Source: CAD feature listing. Evaluate the final solid. Frame: model axes, mm. A direction names the side the tool comes from. Round coordinates to 2 decimals unless told otherwise and drop trailing zeros. Loops run counter-clockwise (first coordinate to the right, second up) from the corner with the lowest first, then second, coordinate; pieces in that order, holes last. Notation, with made-up numbers: (83, 55.25) - (105, 55.25) arc R18 cw to (105, 72.25) - close; hole circle Ø8 at (77.25, 67). An arc over 180 degrees is marked (long way). Use CSV: the item, a comma, the result in double quotes. Start each with the question number.
from build123d import *

# Parameters (mm, degrees)
F0_W     = 86
F0_H     = 66
F1_DEPTH = 2
F2_DEPTH = 10
F3_W     = 92
F3_H     = 72
F3_W_2   = 86
F3_H_2   = 66
F4_DEPTH = 4
F5_W     = 94
F5_H     = 74
F5_W_2   = 88
F5_H_2   = 2
F5_W_3   = 2
F5_H_3   = 68
F6_DEPTH = 2
F0_R     = 2.5
F7_DEPTH = 5


with BuildPart() as f1:
    # F0 (on Top) → F1 (new body)
    with BuildSketch(Plane.XY):
        Rectangle(F0_W, F0_H)
    extrude(amount=F1_DEPTH)

    # F0 (on Top) → F2 (join)
    with BuildSketch(Plane.XY):
        Polygon((47, -37), (47, 37), (5, 37), (-5, 37), (-47, 37), (-47, -37), align=None)
        Rectangle(F0_W, F0_H, mode=Mode.SUBTRACT)
    extrude(amount=F2_DEPTH)

    # F3 (on face) → F4 (cut)
    with BuildSketch(Plane.XY.offset(10)):
        Rectangle(F3_W, F3_H)
        Rectangle(F3_W_2, F3_H_2, mode=Mode.SUBTRACT)
    extrude(amount=-F4_DEPTH, mode=Mode.SUBTRACT)

    # F5 (on face) → F6 (join)
    with BuildSketch(Plane.XY.offset(10)):
        Rectangle(F5_W, F5_H)
        Polygon((-44, -36), (-46, -36), (-46, -34), (-46, 34), (-46, 36), (-44, 36), (44, 36), (46, 36), (46, 34), (46, -34), (46, -36), (44, -36), align=None, mode=Mode.SUBTRACT)
        with Locations((0, 35)):
            Rectangle(F5_W_2, F5_H_2)
        with Locations((0, -35)):
            Rectangle(F5_W_2, F5_H_2)
        with Locations((-45, 0)):
            Rectangle(F5_W_3, F5_H_3)
        with Locations((45, 0)):
            Rectangle(F5_W_3, F5_H_3)
        with Locations((-45, 35)):
            Rectangle(F5_W_3, F5_H_2)
        with Locations((45, 35)):
            Rectangle(F5_W_3, F5_H_2)
        with Locations((45, -35)):
            Rectangle(F5_W_3, F5_H_2)
        with Locations((-45, -35)):
            Rectangle(F5_W_3, F5_H_2)
    extrude(amount=F6_DEPTH)

    # F0 (on Top) → F7 (join)
    with BuildSketch(Plane.XY):
        with BuildLine():
            Line((-5, 37), (5, 37))
            Line((5, 37), (5, 47))
            ThreePointArc((5, 47), (0, 42), (-5, 47))
            Line((-5, 47), (-5, 37))
        make_face()
        with BuildLine():
            ThreePointArc((-5, 47), (0, 42), (5, 47))
            ThreePointArc((5, 47), (0, 52), (-5, 47))
        make_face()
        with Locations((0, 47)):
            Circle(F0_R, mode=Mode.SUBTRACT)
    extrude(amount=F7_DEPTH)


solid = f1.part
1. Section query A-A on x = 0. Return the cut outline in (y, z), and give its area (3 significant figures).
2. Section query D-D on x = 34.5. Return the cut outline in (y, z).
3. Reachability of faces 4 (the flat face through (-1, 33, 4)), 5 (the flat face through (5, 42, 2)), 6 (the flat face through (-5, 42, 2)) from +Z, -Z, +X, -X, +Y, -Y: full face, straight path, thin tool, end or side. Return the list, or none.
4. Contact query for flat-ended pins moving along their axis: P1, Ø4, axis at x = -23, y = 40, coming from the +Z side; P2, Ø0.6, axis at x = -14.5, z = 11.5, coming from the +Y side; P3, Ø1.5, axis at y = 42.5, z = 2.5, coming from the -X side. Output: stop coordinate, or through.
5. Section query C-C on y = -18. Return the cut outline in (x, z).
6. Line query: line 1 along X through (y, z) = (-13.5, 5); line 2 along Y through (x, z) = (7, 7.5); line 3 along X through (y, z) = (16.5, 11). Output: solid intervals per line, ascending.
7. Section query B-B on z = 7.25. Return the cut outline in (x, y).
8. Mould query, pull axis Z, two halves, no side actions, for faces 1 (the flat face through (0, 43, 5)), 2 (the flat face through (-1, -33, 4)), 3 (the flat face through (-1, -36, 8)). Classes: +Z half, -Z half, draft (parallel to the pull), parting line (faces both ways), or undercut.
Values:
1,outline,"(-37, 0) - (44.5, 0) - (44.5, 5) - (37, 5) - (37, 12) - (34, 12) - (34, 10) - (36, 10) - (36, 6) - (33, 6) - (33, 2) - (-33, 2) - (-33, 6) - (-36, 6) - (-36, 10) - (-34, 10) - (-34, 12) - (-37, 12) - close; (49.5, 0) - (52, 0) - (52, 5) - (49.5, 5) - close"
1,area,"250 mm^2"
2,outline,"(-37, 0) - (37, 0) - (37, 12) - (34, 12) - (34, 10) - (36, 10) - (36, 6) - (33, 6) - (33, 2) - (-33, 2) - (-33, 6) - (-36, 6) - (-36, 10) - (-34, 10) - (-34, 12) - (-37, 12) - close"
3,face 4,"+Z"
3,face 5,"+Z, -Z, +X, +Y"
3,face 6,"+Z, -Z, -X, +Y"
4,P1,"passes through"
4,P2,"stops at y = 37"
4,P3,"stops at x = -5"
5,outline,"(-47, 0) - (47, 0) - (47, 12) - (44, 12) - (44, 10) - (46, 10) - (46, 6) - (43, 6) - (43, 2) - (-43, 2) - (-43, 6) - (-46, 6) - (-46, 10) - (-44, 10) - (-44, 12) - (-47, 12) - close"
6,line 1,"x = -47 to -43, 43 to 47"
6,line 2,"y = -37 to -36, 36 to 37"
6,line 3,"x = -47 to -44, 44 to 47"
7,outline,"(-47, -37) - (47, -37) - (47, 37) - (-47, 37) - close; hole (-46, -36) - (46, -36) - (46, 36) - (-46, 36) - close"
8,face 1,"+Z half"
8,face 2,"draft"
8,face 3,"undercut"
